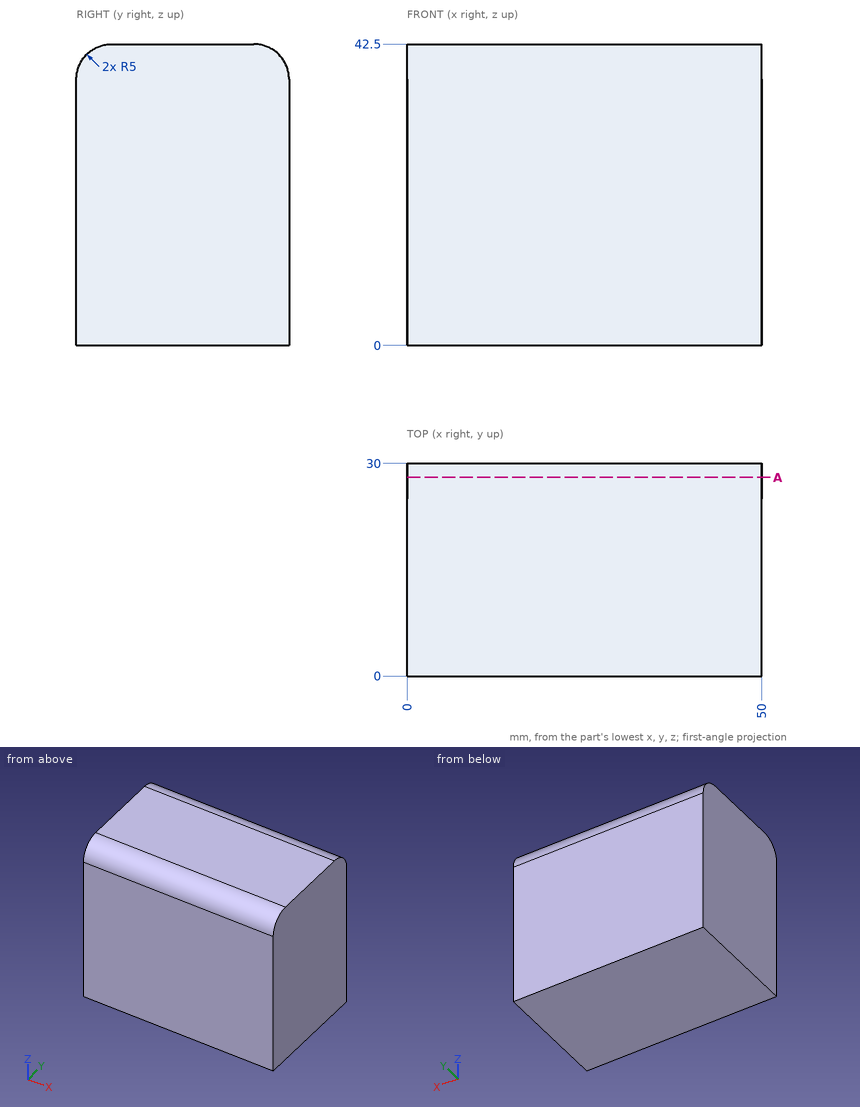
Check sheet for the drawn part. Datum: minimum x, y, z corner. Units: mm. Round coordinates to 2 decimals unless told otherwise and drop trailing zeros. Loops run counter-clockwise (first coordinate to the right, second up) from the corner with the lowest first, then second, coordinate; pieces in that order, holes last. Notation, with made-up numbers: (2, 16) - (27, 16) arc R12 ccw to (27, 23) - close; hole circle Ø4 at (79, 80.5). An arc over 180 degrees is marked (long way). Write each question's results on one line, items separated by ' | '. Start each with the question number.
Q1. Gauge pin test, flat end, axial feed: P1, Ø6, axis at y = 24, z = 6, coming from the -X side. Record the tip position at first contact, or that the pin passes through.
Q2. Cross-section at A-A on y = 28. Enter the section's corners in (x, z), and give its area (4 significant figures).
Q3. Thickness scan on line 1 (Z direction, x = 36.5, y = 25.5); line 2 (Z direction, x = 12, y = 3.75); line 3 (Y direction, x = 13.5, z = 41.5). Record the ranges inside material, lowest first. Write a range as [from, to].
Answers below:
1) P1: stops at x = 0
2) outline: (0, 0) - (50, 0) - (50, 41.5) - (0, 41.5) - close | area: 2,075 mm²
3) line 1: z = [0, 42.47] | line 2: z = [0, 42.34] | line 3: y = [2, 28]
